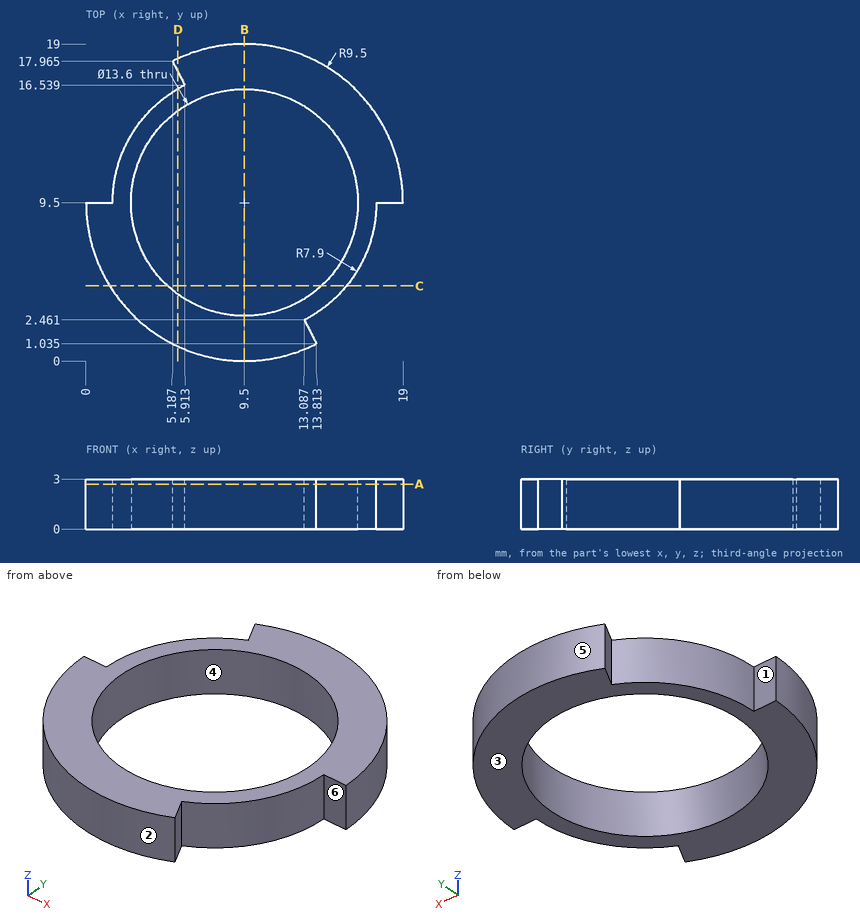
Design review of the part shown in the three views and the two pictorial views. Dimensions are in mm from the part's minimum x, y and z. A direction names the side the tool comes from. Give positions to 0.01 mm unless a question says otherwise; leave off trailing zeros. Loops run counter-clockwise (first coordinate to the right, second up) from the corner with the lowest first, then second, coordinate; pieces in that order, holes last. Notation, with made-up numbers: (27, 65) -> (84, 65) arc R22 ccw to (84, 79) -> close; hole circle Ø2 at (64.5, 66). An arc over 180 degrees is marked (long way). Answer as a JSON object with one key per item and string values. Group by question number.
Q1. Draft analysis for pull direction Y (two halves, no side actions). For the marked faces 1, 2, 3 and 4, state which applies: pulls with the +Y half, pulls with the -Y half, needs draft (parallel to the pull), parting line crosses it, or undercut.
Q2. Wall thickness on line 1 along Y through (x, z) = (9.75, 0.6) (1 decimal); line 2 along X through (y, z) = (9.25, 0.25) (1 decimal); line 3 along Y through (x, z) = (12.5, 0.45) (1 decimal): over which ranges is each line inside the solid? List them lowest first.
Q3. Take a section at C-C (y = 4.5). Write out the cut boundary in (x, z).
Q4. Take a section at A-A (z = 2.7). Write out the cut boundary in (x, y) (1 decimal).
Q5. Tool access review of the marked faces 5 and 6: name each direction out of +Z, -Z, +X, -X, +Y, -Y from which nothing blocks a thin tool from reaching the whole face with its end or side.
Q6. Insertion check: pin 1 (1 mm diameter, centred on x = 15, y = 7, fed in from -Z); pin 2 (1.3 mm diameter, centred on x = 0.5, z = 1, fed in from +Y); pin 3 (1 mm diameter, centred on y = 16.5, z = 2, fed in from +X); pin 4 (1 mm diameter, centred on x = 2.5, z = 1.5, fed in from -Y). Each pin has a flat end and moves straight along its axis. Give the tip position at first contact, or say it passes through.
Q7. Take a section at B-B (x = 9.5). Write out the cut boundary in (y, z).
Q8. Take a section at D-D (x = 5.5). Write out the cut boundary in (y, z), plus the area to 3 significant figures.
Answer below:
{
 "1": {"face 1": "pulls with the +Y half", "face 2": "pulls with the -Y half", "face 3": "needs draft", "face 4": "undercut"},
 "2": {"line 1": "y = 0 to 2.7, 16.3 to 19", "line 2": "x = 0 to 2.7, 16.3 to 17.4", "line 3": "y = 0.5 to 3.4, 15.6 to 18.5"},
 "3": {"outline": "(1.42, 0) -> (4.89, 0) -> (4.89, 3) -> (1.42, 3) -> close; (14.11, 0) -> (15.62, 0) -> (15.62, 3) -> (14.11, 3) -> close"},
 "4": {"outline": "(0, 9.5) arc R9.5 ccw to (13.8, 1) -> (13.1, 2.5) arc R7.9 ccw to (17.4, 9.5) -> (19, 9.5) arc R9.5 ccw to (5.2, 18) -> (5.9, 16.5) arc R7.9 ccw to (1.6, 9.5) -> close; hole circle Ø13.6 at (9.5, 9.5)"},
 "5": {"face 5": "+Z, -Z, +Y", "face 6": "+Z, -Z, +X, -Y"},
 "6": {"pin 1": "passes through", "pin 2": "stops at y = 9.5", "pin 3": "stops at x = 16.43", "pin 4": "stops at y = 2.57"},
 "7": {"outline": "(0, 0) -> (2.7, 0) -> (2.7, 3) -> (0, 3) -> close; (16.3, 0) -> (19, 0) -> (19, 3) -> (16.3, 3) -> close"},
 "8": {"outline": "(0.88, 0) -> (4, 0) -> (4, 3) -> (0.88, 3) -> close; (15, 0) -> (16.31, 0) -> (16.31, 3) -> (15, 3) -> close; (17.35, 0) -> (18.12, 0) -> (18.12, 3) -> (17.35, 3) -> close", "area": "15.6 mm2"}
}
